from build123d import *

# Parameters (mm, degrees)
SM_BASE_FLANGE_1_DEPTH = 4.5
SKETCH_6_R             = 1.5
CUT_EXTRUDE_1_DEPTH    = 10


# Sheet-metal steps are written as plain solids
with BuildPart() as part:
    # Sketch 1 → 基体-法兰1 (new, symmetric)
    with BuildSketch(Plane.XY):
        with BuildLine():
            Line((0, 0), (0, 32.2634))
            ThreePointArc((0, 32.2634), (0.801531583, 34.198468417), (2.7366, 35))
            Line((2.7366, 35), (15, 35))
            Line((15, 35), (15, 33))
            Line((15, 33), (2.7366, 33))
            ThreePointArc((2.7366, 33), (2.215745145, 32.784254855), (2, 32.2634))
            Line((2, 32.2634), (2, 0))
            Line((2, 0), (0, 0))
        make_face()
    extrude(amount=SM_BASE_FLANGE_1_DEPTH, both=True)

    # 草图6 → 切除-拉伸1 (cut)
    with BuildSketch(Plane.ZY):
        with Locations((2.5, 4.75181822)):
            Circle(SKETCH_6_R)
        with Locations((-2.5, 4.75181822)):
            Circle(SKETCH_6_R)
    extrude(amount=-CUT_EXTRUDE_1_DEPTH, mode=Mode.SUBTRACT)


solid = part.part
Read the model definition and answer for the solid it produces. Units are mm, in the model's axes. A direction names the side the tool comes from. Coordinates: 2 decimals unless noted, no trailing zeros. Loops run counter-clockwise (first coordinate to the right, second up) from the corner with the lowest first, then second, coordinate; pieces in that order, holes last.
Q1. The part is cut by section A-A on z = 2.5. Write down the section's boundary in (x, y).
Q2. The part is cut by section B-B on y = 22. Write down the section's boundary in (x, z), and give its area (3 significant figures).
Q3. Each of these flat-tipped pins is pushed along its axis until it touches: pin 1 Ø1.5 at (x, z) = (12.5, -2.5) entering from -Y; pin 2 Ø4.5 at (y, z) = (23.5, 0) entering from +X. Where does it stop, or does it pass through?
Q4. Consider probe 1 along Y at (x, z) = (13.75, 1.25); probe 2 along X at (y, z) = (30.5, -1.75); probe 3 along Y at (x, z) = (1.4, 2.5). Determine where each line is inside the solid, lowest interval first.
Q5. The mould has two halves that part along Z. Classify faces 3 (the face through (1, 21, 4.5)), 4 (the face through (2, 16, 0)), 5 (the face through (0.99, 3.29, 2.17)): +Z half, -Z half, draft (parallel to the pull), parting line (faces both ways), or undercut.
Q6. Which of the six approach directions +Z, -Z, +X, -X, +Y, -Y give full straight-line access (tool end or side, diameter ignored) to faces 1 (the face through (0, 16, 0)), 2 (the face through (9, 33, 0))?
Q7. The part is cut by section C-C on x = 12.25. Write down the section's boundary in (y, z), and give its area (3 significant figures).
Results below:
1. outline: (0, 0) - (2, 0) - (2, 3.25) - (0, 3.25) - close; (0, 6.25) - (2, 6.25) - (2, 32.26) arc R0.74 cw to (2.74, 33) - (15, 33) - (15, 35) - (2.74, 35) arc R2.74 ccw to (0, 32.26) - close
2. outline: (0, -4.5) - (2, -4.5) - (2, 4.5) - (0, 4.5) - close
2. area: 18.0 mm2
3. pin 1: stops at y = 33
3. pin 2: stops at x = 2
4. probe 1: y = 33 to 35
4. probe 2: x = 0 to 2
4. probe 3: y = 0 to 3.25, 6.25 to 34.65
5. face 3: +Z half
5. face 4: draft
5. face 5: undercut
6. face 1: +Z, -Z, -X, +Y, -Y
6. face 2: +Z, -Z, +X, -Y
7. outline: (33, -4.5) - (35, -4.5) - (35, 4.5) - (33, 4.5) - close
7. area: 18.0 mm2
